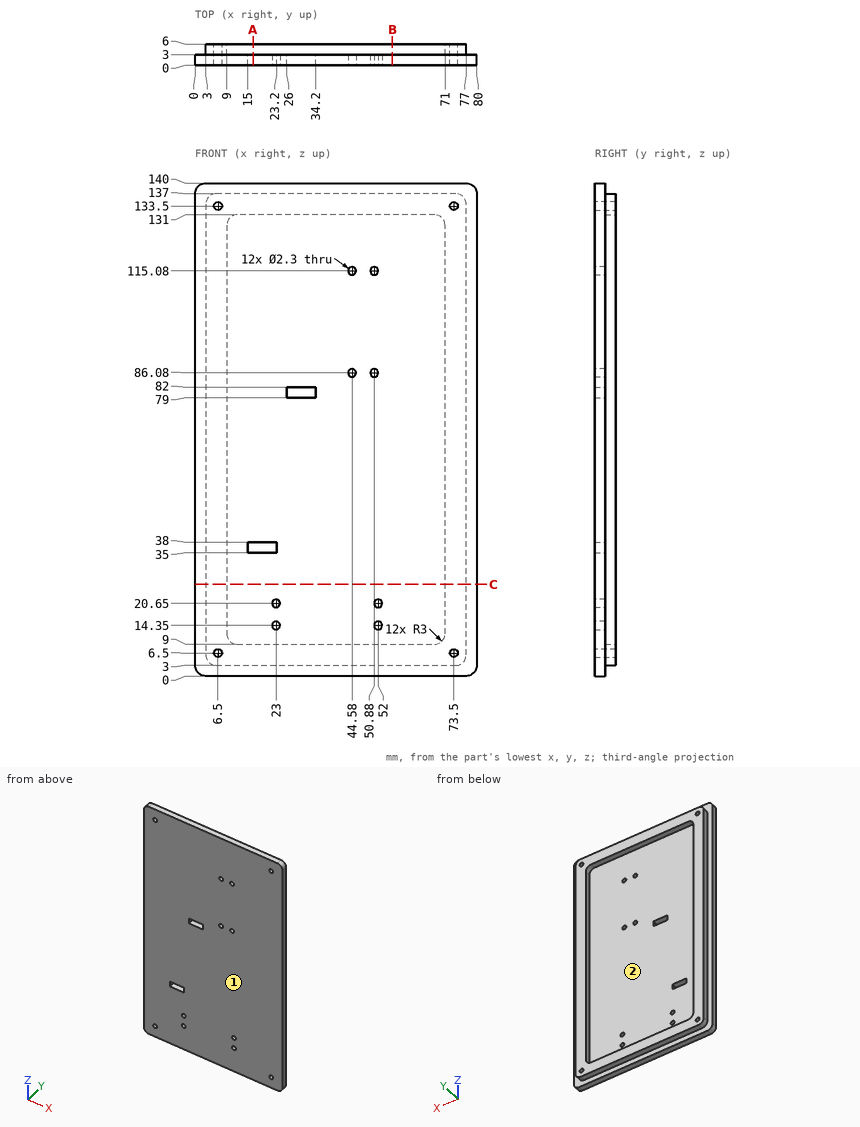
Job drawing, mm, ordinate dimensions from the low corner. One solid piece. Round coordinates to 2 decimals unless told otherwise and drop trailing zeros. Loops run counter-clockwise (first coordinate to the right, second up) from the corner with the lowest first, then second, coordinate; pieces in that order, holes last. Notation, with made-up numbers: (-38, -34.75) -> (11, -34.75) arc R24 ccw to (11, -0.75) -> close; hole circle Ø5 at (-2.75, 51). An arc over 180 degrees is marked (long way). One line per item, written item: value. Start each with the question number.
Q1. Cut at A-A on x = 16.5. List the corners of the cut face in (y, z).
Q2. Probe line 1 along X through (y, z) = (1.35, 115.08); line 2 along X through (y, z) = (3.75, 6.5); line 3 along X through (y, z) = (4.05, 30). List the from-to ranges inside material, lowest first.
Q3. Cut at B-B on x = 56. List the corners of the cut face in (y, z).
Q4. Drop flat-ended pins along their axis: pin 1 Ø2.5 at (x, y) = (17.5, 1.5) entering from -Z; pin 2 Ø0.9 at (x, y) = (38.5, 4.5) entering from -Z; pin 3 Ø1 at (y, z) = (4.5, 60.5) entering from -X; pin 4 Ø3.5 at (x, z) = (50.88, 86.08) entering from +Y. Give the stop position or say it passes through.
Q5. Two-plate mould, pull along Z, no slides. Class the marked faces 1 and 2: released by +Z, released by -Z, zero draft, split by the parting line, or undercut.
Q6. Cut at C-C on z = 26. List the corners of the cut face in (x, y).
Computed:
1. outline: (0, 0) -> (3, 0) -> (3, 3) -> (6, 3) -> (6, 9) -> (3, 9) -> (3, 35) -> (0, 35) -> close; (0, 38) -> (3, 38) -> (3, 131) -> (6, 131) -> (6, 137) -> (3, 137) -> (3, 140) -> (0, 140) -> close
2. line 1: 0 to 43.43, 45.73 to 49.73, 52.03 to 80
2. line 2: 3 to 5.35, 7.65 to 72.35, 74.65 to 77
2. line 3: 3 to 9, 71 to 77
3. outline: (0, 0) -> (3, 0) -> (3, 3) -> (6, 3) -> (6, 9) -> (3, 9) -> (3, 131) -> (6, 131) -> (6, 137) -> (3, 137) -> (3, 140) -> (0, 140) -> close
4. pin 1: z = 0
4. pin 2: z = 3
4. pin 3: x = 3
4. pin 4: y = 3
5. face 1: zero draft
5. face 2: undercut
6. outline: (0, 0) -> (80, 0) -> (80, 3) -> (77, 3) -> (77, 6) -> (71, 6) -> (71, 3) -> (9, 3) -> (9, 6) -> (3, 6) -> (3, 3) -> (0, 3) -> close
